```python
from build123d import *

# Parameters (mm, degrees)
EXTRUDE1_DEPTH          = 9.525
EXTRUDE1_DEPTH_BACK     = 9.525
SKETCH1_R               = 1.4224
SKETCH8_OUTSIDE_W       = 84.186
SKETCH8_OUTSIDE_H       = 85.168
SKETCH8_OUTSIDE_R       = 3.175
EXTRUDE4_DEPTH          = 20.657669199
EXTRUDE4_DRAFT          = -60
MIRROR1_COPY_1_SKETCH_W = 84.186
MIRROR1_COPY_1_SKETCH_H = 85.168
MIRROR1_COPY_1_SKETCH_R = 3.175
MIRROR1_COPY_1_DEPTH    = 20.657669199
MIRROR1_COPY_1_DRAFT    = -60


with BuildPart() as part:
    # Sketch1 → Extrude1 (new, two sides: drawn at the far end of the back side and taken through both)
    with BuildSketch(Plane.XY.offset(-EXTRUDE1_DEPTH_BACK)):
        Polygon((0, 3.666174209), (-3.175, 1.833087105), (-3.175, -1.833087105), (0, -3.666174209), (3.175, -1.833087105), (3.175, 1.833087105), align=None)
        with Locations(Location((0, 0, 0), (0, 0, 180))):
            Circle(SKETCH1_R, mode=Mode.SUBTRACT)
    extrude(amount=EXTRUDE1_DEPTH + EXTRUDE1_DEPTH_BACK)

    # Extrude3 cone 1 section (through the dimple's axis) → Extrude3 (revolve, cut)
    with BuildSketch(Plane(origin=(0, 0, -9.525), x_dir=(0, 1, 0), z_dir=(1, 0, 0))):
        Polygon((0, 0), (1.4732, 0), (0, 1.579813584), align=None)
    extrude3 = revolve(axis=Axis((0, 0, -9.525), (0, 0, 1)), mode=Mode.SUBTRACT)


with BuildPart() as extrude4_tool:
    # Sketch8 outside → Extrude4 (with draft: the straight prism first)
    with BuildSketch(Plane(origin=(0, 0, -9.525), x_dir=(-1, 0, 0), z_dir=(0, 0, -1))):
        Rectangle(SKETCH8_OUTSIDE_W, SKETCH8_OUTSIDE_H)
        Circle(SKETCH8_OUTSIDE_R, mode=Mode.SUBTRACT)
    extrude(amount=-EXTRUDE4_DEPTH)
    # Extrude4: the draft: its side faces are tilted about the plane it starts from
    extrude4_sides = [extrude4_tool.faces().sort_by_distance(p)[0] for p in [
        (0, -42.584, 0.803834599),
        (-42.093, 0, 0.803834599),
        (0, 42.584, 0.803834599),
        (42.093, 0, 0.803834599),
        (3.175, 0, 0.803834599),
    ]]
    draft(extrude4_sides, Plane(origin=(0, 0, -9.525), x_dir=(-1, 0, 0), z_dir=(0, 0, -1)), EXTRUDE4_DRAFT)


with BuildPart() as part_1:
    add(part.part)

    # Extrude4: cut by extrude4_tool
    add(extrude4_tool.part, mode=Mode.SUBTRACT)

    # Mirror1: Extrude3 across plane
    add(extrude3.mirror(Plane.XY), mode=Mode.SUBTRACT)


with BuildPart() as mirror1_copy_1_tool:
    # Mirror1 copy 1 sketch → Mirror1 copy 1 (with draft: the straight prism first)
    with BuildSketch(Plane(origin=(0, 0, 9.525), x_dir=(-1, 0, 0), z_dir=(0, 0, 1))):
        Rectangle(MIRROR1_COPY_1_SKETCH_W, MIRROR1_COPY_1_SKETCH_H)
        Circle(MIRROR1_COPY_1_SKETCH_R, mode=Mode.SUBTRACT)
    extrude(amount=-MIRROR1_COPY_1_DEPTH)
    # Mirror1 copy 1: the draft: its side faces are tilted about the plane it starts from
    mirror1_copy_1_sides = [mirror1_copy_1_tool.faces().sort_by_distance(p)[0] for p in [
        (0, -42.584, -0.803834599),
        (-42.093, 0, -0.803834599),
        (0, 42.584, -0.803834599),
        (42.093, 0, -0.803834599),
        (3.175, 0, -0.803834599),
    ]]
    draft(mirror1_copy_1_sides, Plane(origin=(0, 0, 9.525), x_dir=(-1, 0, 0), z_dir=(0, 0, 1)), MIRROR1_COPY_1_DRAFT)


with BuildPart() as part_2:
    add(part_1.part)

    # Mirror1 copy 1: cut by mirror1_copy_1_tool
    add(mirror1_copy_1_tool.part, mode=Mode.SUBTRACT)


solid = part_2.part
```
For this review, take the finished solid that the model builds, in its own axes (mm). Coordinates: 2 decimals unless noted, no trailing zeros. Write each loop counter-clockwise with the first axis right and the second up, starting at its lowest first coordinate (ties: lowest second). Pieces come first, ordered by that corner, then holes.
(1) The part is to be moulded in two halves that separate along Y. For faces 1 (the face through (0.008, -3.347, -9.426)), 2 (the face through (-0.66, 1.26, -0.13)), 3 (the face through (1.61, 2.737, -0.133)), say which applies: +Y half, -Y half, draft (parallel to the pull), parting line (faces both ways), or undercut.
(2) For pin 1 Ø2.5 at (x, y) = (0, 0) entering from +Z; pin 2 Ø1.5 at (x, y) = (0.5, -1) entering from +Z (3 decimals), all flat-tipped, find the tip position at first contact; note any pin that passes through.
(3) Add section A-A on z = -3. Give the boundary of the cut face in (x, y) (3 decimals).
(4) Wall thickness on probe 1 along Y at (x, z) = (0.25, 1.75); probe 2 along X at (y, z) = (-1.25, 3) (3 decimals); probe 3 along X at (y, z) = (-3, 8.5): over which ranges is each line inside the solid? List them lowest first.
Answer sheet:
1. face 1: -Y half
1. face 2: undercut
1. face 3: +Y half
2. pin 1: passes through
2. pin 2: stops at z = 9.525
3. outline: (-3.175, -1.833) - (0, -3.666) - (3.175, -1.833) - (3.175, 1.833) - (0, 3.666) - (-3.175, 1.833) - close; hole circle Ø2.845 at (0, 0)
4. probe 1: y = -3.52 to -1.4, 1.4 to 3.52
4. probe 2: x = -3.175 to -0.679, 0.679 to 3.175
4. probe 3: x = -1.15 to 1.15
